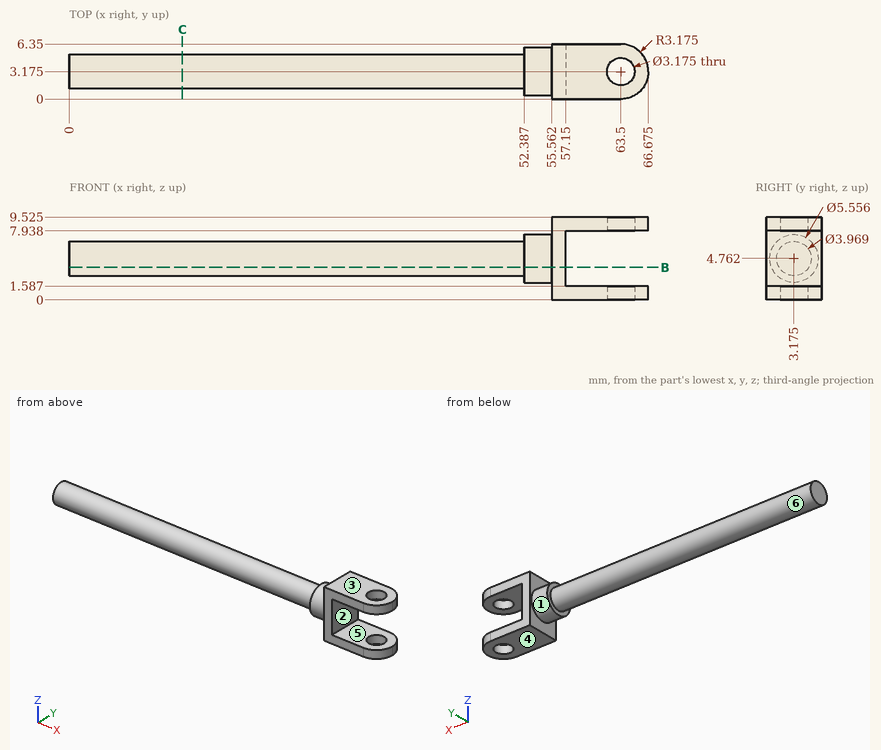
Verification items for this drawing (mm, ordinates from the low corner). A direction names the side the tool comes from. Coordinates: 2 decimals unless noted, no trailing zeros. Write each loop counter-clockwise with the first axis right and the second up, starting at its lowest first coordinate (ties: lowest second). Pieces come first, ordered by that corner, then holes. Notation, with made-up numbers: M 65,46.25 L 70,46.25 A23 cw 70,75.25 Z; hole C -11,17.5 d10. An arc over 180 degrees is marked long. One line per item, written item: value. Start each with the question number.
(1) Release check for a two-part mould opening along Z. For the marked faces 4, 5 and 6 record: released by +Z, released by -Z, zero draft, split by the parting line, or undercut.
(2) Depth check by flat-ended pin: pin 1 (2 mm diameter, centred on x = 37, y = 2.5, fed in from -Z); pin 2 (1.5 mm diameter, centred on y = 5, z = 2, fed in from -X); pin 3 (2 mm diameter, centred on x = 46, y = 3, fed in from +Z); pin 4 (2.5 mm diameter, centred on x = 63.5, y = 3.175, fed in from -Z). Enter the tip coordinate at first touch or a pass-through.
(3) Sectioned sample at B-B, the plane z = 3.75. Enter the section's corners in (x, y), and give its area (3 significant figures).
(4) Tool access check on the marked faces 1, 2 and 3. Record the directions out of +Z, -Z, +X, -X, +Y, -Y that give a thin tool (end or side, any length) a straight path to the whole face; none if there is none.
(5) Sectioned sample at C-C, the plane x = 13. Enter the section's corners in (y, z) (1 decimal).
(6) Scan lines: line 1 along Y through (x, z) = (63.5, 8.3); line 2 along Z through (x, y) = (64.5, 1.75) (1 decimal); line 3 along X through (y, z) = (5.5, 5.75). Record each from-to range of solid material in increasing order. Write a range as [from, to].
Filled sheet:
1. face 4: released by -Z
1. face 5: undercut
1. face 6: split by the parting line
2. pin 1: z = 2.78
2. pin 2: x = 52.39
2. pin 3: z = 6.75
2. pin 4: through
3. outline: M 0,1.47 L 52.39,1.47 L 52.39,0.59 L 55.56,0.59 L 55.56,0 L 57.15,0 L 57.15,6.35 L 55.56,6.35 L 55.56,5.76 L 52.39,5.76 L 52.39,4.88 L 0,4.88 Z
3. area: 205 mm²
4. face 1: -X
4. face 2: +X, +Y, -Y
4. face 3: +Z, +X, -X, +Y, -Y
5. outline: C 3.2,4.8 d4
6. line 1: [0, 1.59], [4.76, 6.35]
6. line 2: [0, 1.6], [7.9, 9.5]
6. line 3: [52.39, 57.15]
